CAD build for the part. Positions are in the model's coordinates, mm. A direction names the side the tool comes from. Coordinates: 2 decimals unless noted, no trailing zeros. Order: outer loops, then holes, each group sorted by start corner. A loop starts at its lowest first (then second) coordinate and runs counter-clockwise, first axis right, second up. Notation, with made-up numbers: M -3.75,-6 L 42.25,-6 A27 cw 42.25,18 Z; hole C 42.5,54.25 d7. An arc over 180 degrees is marked long. Write item = value, one per line.
from build123d import *

# Parameters (mm, degrees)
F0_W     = 26
F0_H     = 7.1
F0_R     = 4
F1_DEPTH = 10
F2_DEPTH = 1.2
F3_DEPTH = 4.2


# Not quite as in the source:
# - a feature names something its author has since deleted; it is built from what else it names


with BuildPart() as f1:
    # F0 (on Top) → F1 (new body)
    with BuildSketch(Plane.XY):
        with BuildLine():
            Line((-20, -60), (20, -60))
            Line((20, -60), (20, 60))
            Line((20, 60), (-20, 60))
            Line((-20, 60), (-20, 25.55))
            Line((-20, 25.55), (-1.2083045974, 25.55))
            ThreePointArc((-1.2083045974, 25.55), (2.1830434902, 25.0490688939), (3.75, 22))
            ThreePointArc((3.75, 22), (2.1830434902, 18.9509311061), (-1.2083045974, 18.45))
            Line((-1.2083045974, 18.45), (-20, 18.45))
            Line((-20, 18.45), (-20, 11.55))
            Line((-20, 11.55), (-1.2083045974, 11.55))
            ThreePointArc((-1.2083045974, 11.55), (2.1830434902, 11.0490688939), (3.75, 8))
            ThreePointArc((3.75, 8), (2.1830434902, 4.9509311061), (-1.2083045974, 4.45))
            Line((-1.2083045974, 4.45), (-20, 4.45))
            Line((-20, 4.45), (-20, -4.45))
            Line((-20, -4.45), (-1.2083045974, -4.45))
            ThreePointArc((-1.2083045974, -4.45), (2.1830434902, -4.9509311061), (3.75, -8))
            ThreePointArc((3.75, -8), (2.1830434902, -11.0490688939), (-1.2083045974, -11.55))
            Line((-1.2083045974, -11.55), (-20, -11.55))
            Line((-20, -11.55), (-20, -18.45))
            Line((-20, -18.45), (-1.2083045974, -18.45))
            ThreePointArc((-1.2083045974, -18.45), (2.1830434902, -18.9509311061), (3.75, -22))
            ThreePointArc((3.75, -22), (2.1830434902, -25.0490688939), (-1.2083045974, -25.55))
            Line((-1.2083045974, -25.55), (-20, -25.55))
            Line((-20, -25.55), (-20, -60))
        make_face()
        with Locations((-4, -37.95)):
            Rectangle(F0_W, F0_H, mode=Mode.SUBTRACT)
        with Locations((0, -50)):
            Circle(F0_R, mode=Mode.SUBTRACT)
        with Locations((-4, 37.95)):
            Rectangle(F0_W, F0_H, mode=Mode.SUBTRACT)
        with Locations((0, 50)):
            Circle(F0_R, mode=Mode.SUBTRACT)
        with BuildLine():
            Line((-20, -18.45), (-20, -25.55))
            Line((-20, -25.55), (-1.2083045974, -25.55))
            ThreePointArc((-1.2083045974, -25.55), (-3.75, -22), (-1.2083045974, -18.45))
            Line((-1.2083045974, -18.45), (-20, -18.45))
        make_face()
        with BuildLine():
            Line((-1.2083045974, 25.55), (-20, 25.55))
            Line((-20, 25.55), (-20, 18.45))
            Line((-20, 18.45), (-1.2083045974, 18.45))
            ThreePointArc((-1.2083045974, 18.45), (-3.75, 22), (-1.2083045974, 25.55))
        make_face()
        with BuildLine():
            Line((-20, -4.45), (-20, -11.55))
            Line((-20, -11.55), (-1.2083045974, -11.55))
            ThreePointArc((-1.2083045974, -11.55), (-3.75, -8), (-1.2083045974, -4.45))
            Line((-1.2083045974, -4.45), (-20, -4.45))
        make_face()
        with BuildLine():
            Line((-1.2083045974, 11.55), (-20, 11.55))
            Line((-20, 11.55), (-20, 4.45))
            Line((-20, 4.45), (-1.2083045974, 4.45))
            ThreePointArc((-1.2083045974, 4.45), (-3.75, 8), (-1.2083045974, 11.55))
        make_face()
        with BuildLine():
            Line((0, 25.55), (-1.2083045974, 25.55))
            ThreePointArc((-1.2083045974, 25.55), (-3.75, 22), (-1.2083045974, 18.45))
            Line((-1.2083045974, 18.45), (0, 18.45))
            Line((0, 18.45), (0, 20.25))
            ThreePointArc((0, 20.25), (-1.75, 22), (0, 23.75))
            Line((0, 23.75), (0, 25.55))
        make_face()
        with BuildLine():
            ThreePointArc((3.75, 22), (2.1830434902, 25.0490688939), (-1.2083045974, 25.55))
            Line((-1.2083045974, 25.55), (0, 25.55))
            Line((0, 25.55), (0, 23.75))
            ThreePointArc((0, 23.75), (1.2374368671, 23.2374368671), (1.75, 22))
            ThreePointArc((1.75, 22), (1.2374368671, 20.7625631329), (0, 20.25))
            Line((0, 20.25), (0, 18.45))
            Line((0, 18.45), (-1.2083045974, 18.45))
            ThreePointArc((-1.2083045974, 18.45), (2.1830434902, 18.9509311061), (3.75, 22))
        make_face()
        with BuildLine():
            ThreePointArc((3.75, 8), (2.1830434902, 11.0490688939), (-1.2083045974, 11.55))
            Line((-1.2083045974, 11.55), (0, 11.55))
            Line((0, 11.55), (0, 9.75))
            ThreePointArc((0, 9.75), (1.2374368671, 9.2374368671), (1.75, 8))
            ThreePointArc((1.75, 8), (1.2374368671, 6.7625631329), (0, 6.25))
            Line((0, 6.25), (0, 4.45))
            Line((0, 4.45), (-1.2083045974, 4.45))
            ThreePointArc((-1.2083045974, 4.45), (2.1830434902, 4.9509311061), (3.75, 8))
        make_face()
        with BuildLine():
            Line((0, 11.55), (-1.2083045974, 11.55))
            ThreePointArc((-1.2083045974, 11.55), (-3.75, 8), (-1.2083045974, 4.45))
            Line((-1.2083045974, 4.45), (0, 4.45))
            Line((0, 4.45), (0, 6.25))
            ThreePointArc((0, 6.25), (-1.75, 8), (0, 9.75))
            Line((0, 9.75), (0, 11.55))
        make_face()
        with BuildLine():
            ThreePointArc((-1.2083045974, -4.45), (-3.75, -8), (-1.2083045974, -11.55))
            Line((-1.2083045974, -11.55), (0, -11.55))
            Line((0, -11.55), (0, -9.75))
            ThreePointArc((0, -9.75), (-1.75, -8), (0, -6.25))
            Line((0, -6.25), (0, -4.45))
            Line((0, -4.45), (-1.2083045974, -4.45))
        make_face()
        with BuildLine():
            Line((0, -11.55), (-1.2083045974, -11.55))
            ThreePointArc((-1.2083045974, -11.55), (2.1830434902, -11.0490688939), (3.75, -8))
            ThreePointArc((3.75, -8), (2.1830434902, -4.9509311061), (-1.2083045974, -4.45))
            Line((-1.2083045974, -4.45), (0, -4.45))
            Line((0, -4.45), (0, -6.25))
            ThreePointArc((0, -6.25), (1.2374368671, -6.7625631329), (1.75, -8))
            ThreePointArc((1.75, -8), (1.2374368671, -9.2374368671), (0, -9.75))
            Line((0, -9.75), (0, -11.55))
        make_face()
        with BuildLine():
            Line((0, -25.55), (-1.2083045974, -25.55))
            ThreePointArc((-1.2083045974, -25.55), (2.1830434902, -25.0490688939), (3.75, -22))
            ThreePointArc((3.75, -22), (2.1830434902, -18.9509311061), (-1.2083045974, -18.45))
            Line((-1.2083045974, -18.45), (0, -18.45))
            Line((0, -18.45), (0, -20.25))
            ThreePointArc((0, -20.25), (1.2374368671, -20.7625631329), (1.75, -22))
            ThreePointArc((1.75, -22), (1.2374368671, -23.2374368671), (0, -23.75))
            Line((0, -23.75), (0, -25.55))
        make_face()
        with BuildLine():
            ThreePointArc((-1.2083045974, -18.45), (-3.75, -22), (-1.2083045974, -25.55))
            Line((-1.2083045974, -25.55), (0, -25.55))
            Line((0, -25.55), (0, -23.75))
            ThreePointArc((0, -23.75), (-1.75, -22), (0, -20.25))
            Line((0, -20.25), (0, -18.45))
            Line((0, -18.45), (-1.2083045974, -18.45))
        make_face()
        with Locations((-4, 37.95)):
            Rectangle(F0_W, F0_H)
        with Locations((-4, -37.95)):
            Rectangle(F0_W, F0_H)
    extrude(amount=-F1_DEPTH)

    # F0 (on Top) → F2 (cut)
    with BuildSketch(Plane.XY):
        with BuildLine():
            Line((-1.2083045974, 25.55), (-20, 25.55))
            Line((-20, 25.55), (-20, 18.45))
            Line((-20, 18.45), (-1.2083045974, 18.45))
            ThreePointArc((-1.2083045974, 18.45), (-3.75, 22), (-1.2083045974, 25.55))
        make_face()
        with BuildLine():
            Line((-1.2083045974, 11.55), (-20, 11.55))
            Line((-20, 11.55), (-20, 4.45))
            Line((-20, 4.45), (-1.2083045974, 4.45))
            ThreePointArc((-1.2083045974, 4.45), (-3.75, 8), (-1.2083045974, 11.55))
        make_face()
        with BuildLine():
            Line((-20, -4.45), (-20, -11.55))
            Line((-20, -11.55), (-1.2083045974, -11.55))
            ThreePointArc((-1.2083045974, -11.55), (-3.75, -8), (-1.2083045974, -4.45))
            Line((-1.2083045974, -4.45), (-20, -4.45))
        make_face()
        with BuildLine():
            Line((-20, -18.45), (-20, -25.55))
            Line((-20, -25.55), (-1.2083045974, -25.55))
            ThreePointArc((-1.2083045974, -25.55), (-3.75, -22), (-1.2083045974, -18.45))
            Line((-1.2083045974, -18.45), (-20, -18.45))
        make_face()
        with Locations((-4, 37.95)):
            Rectangle(F0_W, F0_H)
        with Locations((-4, -37.95)):
            Rectangle(F0_W, F0_H)
    extrude(amount=-F2_DEPTH, mode=Mode.SUBTRACT)

    # F0 (on Top) → F3 (cut)
    with BuildSketch(Plane.XY):
        with BuildLine():
            Line((0, 25.55), (-1.2083045974, 25.55))
            ThreePointArc((-1.2083045974, 25.55), (-3.75, 22), (-1.2083045974, 18.45))
            Line((-1.2083045974, 18.45), (0, 18.45))
            Line((0, 18.45), (0, 20.25))
            ThreePointArc((0, 20.25), (-1.75, 22), (0, 23.75))
            Line((0, 23.75), (0, 25.55))
        make_face()
        with BuildLine():
            ThreePointArc((3.75, 22), (2.1830434902, 25.0490688939), (-1.2083045974, 25.55))
            Line((-1.2083045974, 25.55), (0, 25.55))
            Line((0, 25.55), (0, 23.75))
            ThreePointArc((0, 23.75), (1.2374368671, 23.2374368671), (1.75, 22))
            ThreePointArc((1.75, 22), (1.2374368671, 20.7625631329), (0, 20.25))
            Line((0, 20.25), (0, 18.45))
            Line((0, 18.45), (-1.2083045974, 18.45))
            ThreePointArc((-1.2083045974, 18.45), (2.1830434902, 18.9509311061), (3.75, 22))
        make_face()
        with BuildLine():
            Line((0, 11.55), (-1.2083045974, 11.55))
            ThreePointArc((-1.2083045974, 11.55), (-3.75, 8), (-1.2083045974, 4.45))
            Line((-1.2083045974, 4.45), (0, 4.45))
            Line((0, 4.45), (0, 6.25))
            ThreePointArc((0, 6.25), (-1.75, 8), (0, 9.75))
            Line((0, 9.75), (0, 11.55))
        make_face()
        with BuildLine():
            ThreePointArc((3.75, 8), (2.1830434902, 11.0490688939), (-1.2083045974, 11.55))
            Line((-1.2083045974, 11.55), (0, 11.55))
            Line((0, 11.55), (0, 9.75))
            ThreePointArc((0, 9.75), (1.2374368671, 9.2374368671), (1.75, 8))
            ThreePointArc((1.75, 8), (1.2374368671, 6.7625631329), (0, 6.25))
            Line((0, 6.25), (0, 4.45))
            Line((0, 4.45), (-1.2083045974, 4.45))
            ThreePointArc((-1.2083045974, 4.45), (2.1830434902, 4.9509311061), (3.75, 8))
        make_face()
        with BuildLine():
            ThreePointArc((-1.2083045974, -4.45), (-3.75, -8), (-1.2083045974, -11.55))
            Line((-1.2083045974, -11.55), (0, -11.55))
            Line((0, -11.55), (0, -9.75))
            ThreePointArc((0, -9.75), (-1.75, -8), (0, -6.25))
            Line((0, -6.25), (0, -4.45))
            Line((0, -4.45), (-1.2083045974, -4.45))
        make_face()
        with BuildLine():
            Line((0, -11.55), (-1.2083045974, -11.55))
            ThreePointArc((-1.2083045974, -11.55), (2.1830434902, -11.0490688939), (3.75, -8))
            ThreePointArc((3.75, -8), (2.1830434902, -4.9509311061), (-1.2083045974, -4.45))
            Line((-1.2083045974, -4.45), (0, -4.45))
            Line((0, -4.45), (0, -6.25))
            ThreePointArc((0, -6.25), (1.2374368671, -6.7625631329), (1.75, -8))
            ThreePointArc((1.75, -8), (1.2374368671, -9.2374368671), (0, -9.75))
            Line((0, -9.75), (0, -11.55))
        make_face()
        with BuildLine():
            Line((0, -25.55), (-1.2083045974, -25.55))
            ThreePointArc((-1.2083045974, -25.55), (2.1830434902, -25.0490688939), (3.75, -22))
            ThreePointArc((3.75, -22), (2.1830434902, -18.9509311061), (-1.2083045974, -18.45))
            Line((-1.2083045974, -18.45), (0, -18.45))
            Line((0, -18.45), (0, -20.25))
            ThreePointArc((0, -20.25), (1.2374368671, -20.7625631329), (1.75, -22))
            ThreePointArc((1.75, -22), (1.2374368671, -23.2374368671), (0, -23.75))
            Line((0, -23.75), (0, -25.55))
        make_face()
        with BuildLine():
            ThreePointArc((-1.2083045974, -18.45), (-3.75, -22), (-1.2083045974, -25.55))
            Line((-1.2083045974, -25.55), (0, -25.55))
            Line((0, -25.55), (0, -23.75))
            ThreePointArc((0, -23.75), (-1.75, -22), (0, -20.25))
            Line((0, -20.25), (0, -18.45))
            Line((0, -18.45), (-1.2083045974, -18.45))
        make_face()
    extrude(amount=-F3_DEPTH, mode=Mode.SUBTRACT)


solid = f1.part
(1) Slice it at A-A, the plane y = -50. Write the cut outline in (x, z), then the cut area to 3 significant figures.
Evaluation:
outline = M -20,-10 L -4,-10 L -4,0 L -20,0 Z; M 4,-10 L 20,-10 L 20,0 L 4,0 Z
area = 320 mm²
(2) Pin check, flat tips, straight feed: pin 1 Ø2 at (x, y) = (-1, -9.5) entering from +Z; pin 2 Ø3.5 at (x, y) = (-8, 8.5) entering from +Z. Stop position of each tip, or through.
Evaluation:
pin_1 = -4.2
pin_2 = -1.2
(3) Pull direction Y, two halves, no side cores. Call faces 1 (the face through (0, 1, 0)), 2 (the face through (0, -60, -5)), 3 (the face through (1, 6, -4.2)): +Y half, -Y half, draft (parallel to the pull), parting line (faces both ways), or undercut.
Evaluation:
face_1 = draft
face_2 = -Y half
face_3 = undercut
(4) Tool access for faces 4 (the face through (-11, -22, -1.2)), 5 (the face through (-4, -38, -1.2)), 6 (the face through (-0.867, 46.095, -4.93)): list every direction of +Z, -Z, +X, -X, +Y, -Y with a clear straight run to the whole face (end or side of a thin tool).
Evaluation:
face_4 = +Z, -X
face_5 = +Z
face_6 = +Z, -Z
(5) Slice it at C-C, the plane x = -14. Write the cut outline in (y, z), then the cut area to 3 significant figures.
Evaluation:
outline = M -60,-10 L 60,-10 L 60,0 L 41.5,0 L 41.5,-1.2 L 34.4,-1.2 L 34.4,0 L 25.55,0 L 25.55,-1.2 L 18.45,-1.2 L 18.45,0 L 11.55,0 L 11.55,-1.2 L 4.45,-1.2 L 4.45,0 L -4.45,0 L -4.45,-1.2 L -11.55,-1.2 L -11.55,0 L -18.45,0 L -18.45,-1.2 L -25.55,-1.2 L -25.55,0 L -34.4,0 L -34.4,-1.2 L -41.5,-1.2 L -41.5,0 L -60,0 Z
area = 1,150 mm²
(6) Slice it at B-B, the plane z = -5.25. Write the cut outline in (x, y), then the cut area to 3 significant figures.
Evaluation:
outline = M -20,-60 L 20,-60 L 20,60 L -20,60 Z; hole C 0,-50 d8; hole C 0,50 d8; hole C 0,-22 d3.5; hole C 0,-8 d3.5; hole C 0,8 d3.5; hole C 0,22 d3.5
area = 4,660 mm²
(7) Wall check: line 1 (Z direction, x = 2, y = -5); line 2 (Z direction, x = 7.5, y = 40.5). Give the ranges that are in metal, low to high. Write a range as from..to.
Evaluation:
line_1 = -10..-4.2
line_2 = -10..-1.2
